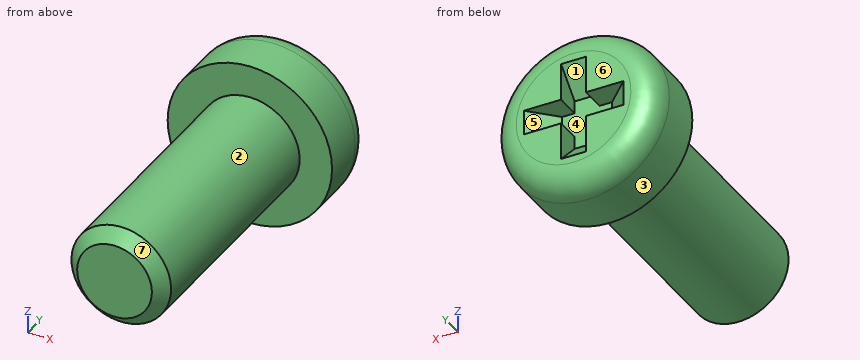
```python
from build123d import *

# Parameters (mm, degrees)
SKETCH_1_R          = 2
EXTRUDE_1_DEPTH     = 10
SKETCH_2_R          = 3.3
EXTRUDE_2_DEPTH     = 2.7
FILLET_1_R          = 1
CHAMFER_1_SIZE      = 0.5
SKETCH_3_W          = 4
SKETCH_3_H          = 1
SKETCH_3_W_2        = 1
SKETCH_3_H_2        = 4
CUT_EXTRUDE_1_DEPTH = 1
CHAMFER_2_SIZE      = 1


with BuildPart() as part:
    # 草图1 → 凸台-拉伸1 (new body)
    with BuildSketch(Plane(origin=(0, 0, 0), x_dir=(1, 0, 0), z_dir=(0, 1, 0))):
        with Locations(Location((0, 0, 0), (0, 0, 270))):
            Circle(SKETCH_1_R)
    extrude(amount=EXTRUDE_1_DEPTH)

    # 草图2 → 凸台-拉伸2 (add)
    with BuildSketch(Plane(origin=(0, 10, 0), x_dir=(1, 0, 0), z_dir=(0, 1, 0))):
        with Locations(Location((0, 0, 0), (0, 0, 90))):
            Circle(SKETCH_2_R)
    extrude(amount=EXTRUDE_2_DEPTH)

    # 圆角1
    fillet_1_edges = [part.edges().sort_by_distance(p)[0] for p in [
        (0, 12.7, 3.3),
    ]]
    fillet(fillet_1_edges, radius=FILLET_1_R)

    # 倒角1
    chamfer_1_edges = [part.edges().sort_by_distance(p)[0] for p in [
        (0, 0, -2),
    ]]
    chamfer(chamfer_1_edges, length=CHAMFER_1_SIZE)

    # 草图3 → 切除-拉伸-薄壁1 (cut)
    with BuildSketch(Plane(origin=(0, 12.7, 0), x_dir=(1, 0, 0), z_dir=(0, 1, 0))):
        Rectangle(SKETCH_3_W, SKETCH_3_H)
        Rectangle(SKETCH_3_W_2, SKETCH_3_H_2)
    extrude(amount=-CUT_EXTRUDE_1_DEPTH, mode=Mode.SUBTRACT)

    # 倒角2
    chamfer_2_edges = [part.edges().sort_by_distance(p)[0] for p in [
        (0, 11.7, 2),
        (2, 11.7, 0),
        (0, 11.7, -2),
        (-2, 11.7, 0),
    ]]
    chamfer(chamfer_2_edges, length=CHAMFER_2_SIZE - 0.0001)  # a hair under: the kernel refuses the full size


solid = part.part
```
Build history of the part. All positions in model axes, mm. Face numbers are marked on the shaded views. A direction names the side the tool comes from. Coordinates: 2 decimals unless noted, no trailing zeros. Order: outer loops, then holes, each group sorted by start corner. A loop starts at its lowest first (then second) coordinate and runs counter-clockwise, first axis right, second up. Notation, with made-up numbers: (-11.75, 72.25) -> (37.25, 72.25) arc R30 cw to (37.25, 97.25) -> close; hole circle Ø6 at (33.25, -29.75). An arc over 180 degrees is marked (long way). Answer in a Markdown table with one row per item. Add a question column.
Q1. Band-saw the part on C-C, the plane y = 7.5. List the corners of the cut face in (x, z), then the cut area to 3 significant figures.
Q2. Drop flat-ended pins along their axis: pin 1 (0.5 mm diameter, centred on x = -1, y = 12.5, fed in from -Z); pin 2 (0.8 mm diameter, centred on y = 12.5, z = -1, fed in from +X); pin 3 (0.8 mm diameter, centred on x = 1.5, y = 12.5, fed in from -Z). Give the stop position or say it passes through.
Q3. Wall check: line 1 along X through (y, z) = (6.5, 0); line 2 along Z through (x, y) = (0.25, 11.75); line 3 along Z through (x, y) = (-0.25, 12). Give the ranges that are in metal, low to high. Write a range as [from, to].
Q4. Which spindle directions (+Z, -Z, +X, -X, +Y, -Y) get a long thin tool onto all of the face, cutting with end or side? Do the marked faces 1, 2 and 3. Say none if no direction does.
Q5. Mould opens along Z. For the marked faces 4, 5, 6 and 7 say: +Z half, -Z half, draft (parallel to the pull), parting line (faces both ways), or undercut.
Answers follow:
| question | item | result |
|---|---|---|
| 1 | outline | circle Ø4 at (0, 0) |
| 1 | area | 12.6 mm^2 |
| 2 | pin 1 | z = -2.99 |
| 2 | pin 2 | x = 3.09 |
| 2 | pin 3 | z = -2.92 |
| 3 | line 1 | [-2, 2] |
| 3 | line 2 | [-3.29, -1.05], [1.05, 3.29] |
| 3 | line 3 | [-3.24, -1.3], [1.3, 3.24] |
| 4 | face 1 | +Y |
| 4 | face 2 | -Y |
| 4 | face 3 | +Y, -Y |
| 5 | face 4 | undercut |
| 5 | face 5 | undercut |
| 5 | face 6 | draft |
| 5 | face 7 | parting line |
